```python
from build123d import *

# Parameters (mm, degrees)
BOSS_EXTRUDE1_DEPTH = 35.7124
FILLET1_R           = 6.35
CUT_EXTRUDE1_DEPTH  = 65.64205685
CUT_EXTRUDE2_REACH  = 66.642
SKETCH4_R           = 4.1656


with BuildPart() as part:
    # Sketch2 → Boss-Extrude1 (new, symmetric)
    with BuildSketch(Plane.XY):
        with BuildLine():
            Line((0, 0), (0, 38.1))
            Line((0, 38.1), (6.35, 38.1))
            Line((6.35, 38.1), (6.35, 14.2748))
            ThreePointArc((6.35, 14.2748), (8.67112018, 8.67112018), (14.2748, 6.35))
            Line((14.2748, 6.35), (38.1, 6.35))
            Line((38.1, 6.35), (38.1, 0))
            Line((38.1, 0), (0, 0))
        make_face()
    extrude(amount=BOSS_EXTRUDE1_DEPTH, both=True)

    # Fillet1
    fillet1_edges = [part.edges().sort_by_distance(p)[0] for p in [
        (38.1, 6.35, 0),
        (6.35, 38.1, 0),
    ]]
    fillet(fillet1_edges, radius=FILLET1_R - 0.0001)  # a hair under: the kernel refuses the full size

    # Sketch3 → Cut-Extrude1 (cut, through all)
    with BuildSketch(Plane.ZY):
        with BuildLine():
            Line((-23.2156, 25.4), (-23.2156, 12.7))
            ThreePointArc((-23.2156, 12.7), (-19.05, 8.5344), (-14.8844, 12.7))
            Line((-14.8844, 12.7), (-14.8844, 25.4))
            ThreePointArc((-14.8844, 25.4), (-19.05, 29.5656), (-23.2156, 25.4))
        make_face()
        with BuildLine():
            Line((14.8844, 12.7), (14.8844, 25.4))
            ThreePointArc((14.8844, 25.4), (19.05, 29.5656), (23.2156, 25.4))
            Line((23.2156, 25.4), (23.2156, 12.7))
            ThreePointArc((23.2156, 12.7), (19.05, 8.5344), (14.8844, 12.7))
        make_face()
    extrude(amount=-CUT_EXTRUDE1_DEPTH, mode=Mode.SUBTRACT)

    # Sketch4 → Cut-Extrude2 (cut, up to next)
    with BuildSketch(Plane.XZ, mode=Mode.PRIVATE) as cut_extrude2_sk1:
        with Locations((19.05, -19.05)):
            Circle(SKETCH4_R)
    cut_extrude2_tool1 = extrude(cut_extrude2_sk1.sketch, amount=-CUT_EXTRUDE2_REACH, mode=Mode.PRIVATE) & part.part
    # Sketch4 → Cut-Extrude2 (cut, up to next)
    with BuildSketch(Plane.XZ, mode=Mode.PRIVATE) as cut_extrude2_sk2:
        with Locations((19.05, 19.05)):
            Circle(SKETCH4_R)
    cut_extrude2_tool2 = extrude(cut_extrude2_sk2.sketch, amount=-CUT_EXTRUDE2_REACH, mode=Mode.PRIVATE) & part.part
    add(cut_extrude2_tool1.solids().sort_by_distance((19.05, 0, -19.05))[0], mode=Mode.SUBTRACT)
    add(cut_extrude2_tool2.solids().sort_by_distance((19.05, 0, 19.05))[0], mode=Mode.SUBTRACT)


solid = part.part
```
CAD build for the part. Positions are in the model's coordinates, mm. A direction names the side the tool comes from. Coordinates: 2 decimals unless noted, no trailing zeros. Order: outer loops, then holes, each group sorted by start corner. A loop starts at its lowest first (then second) coordinate and runs counter-clockwise, first axis right, second up.
(1) Drill centre lines: L1, parallel to Z at x = 19, y = 3; L2, parallel to Y at x = 28, z = 26.5. Where is each one in solid material? Low to high.
Solution:
L1: z = -35.71 to -23.22, -14.88 to 14.88, 23.22 to 35.71
L2: y = 0 to 6.35
(2) Mould opens along Y. For faces 1 (the face through (8.61, 8.733, 0.5)), 2 (the face through (4.344, 8.535, -19.142)), 3 (the face through (11, 6, -35.712)) say: released by +Y, released by -Y, zero draft, split by the parting line, or undercut.
Solution:
face 1: released by +Y
face 2: undercut
face 3: zero draft
(3) Pin check, flat tips, straight feed: pin 1 Ø4 at (y, z) = (22.5, 20) entering from +X; pin 2 Ø1.5 at (x, z) = (19.5, 4.5) entering from +Y; pin 3 Ø14 at (y, z) = (24, -15) entering from +X; pin 4 Ø19 at (x, z) = (19, -1) entering from +Y. Stop position of each tip, or through.
Solution:
pin 1: passes through
pin 2: stops at y = 6.35
pin 3: stops at x = 6.35
pin 4: stops at y = 7.95
(4) Saw through at B-B, the plane z = -19.05. Count the separate pieces of the cut face and the enclosed holes in it, and give its area (3 significant figures).
Solution:
separate pieces: 3
enclosed holes: 0
area: 249 mm2
(5) Saw through at A-A, the plane x = 19.05. Write the cut outline in (y, z), and give its area (3 significant figures).
Solution:
outline: (0, -35.71) - (6.35, -35.71) - (6.35, -23.22) - (0, -23.22) - close; (0, -14.88) - (6.35, -14.88) - (6.35, 14.88) - (0, 14.88) - close; (0, 23.22) - (6.35, 23.22) - (6.35, 35.71) - (0, 35.71) - close
area: 348 mm2
(6) Which spindle directions (+Z, -Z, +X, -X, +Y, -Y) get a long thin tool onto all of the face, cutting with end or side? Do faces 4 (the face through (19, 0, 0)), 5 (the face through (6.35, 23, 0)), 6 (the face through (3, 19, -14.884)). Say none if no direction does.
Solution:
face 4: +Z, -Z, +X, -X, -Y
face 5: +Z, -Z, +X, +Y
face 6: +X, -X
